The model under review builds one solid part; all positions refer to its coordinate system, in mm. A direction names the side the tool comes from. Give positions to 0.01 mm unless a question says otherwise; leave off trailing zeros. Order: outer loops, then holes, each group sorted by start corner. A loop starts at its lowest first (then second) coordinate and runs counter-clockwise, first axis right, second up. Notation, with made-up numbers: (0.25, 4.25) - (43.25, 4.25) arc R30 ccw to (43.25, 39.25) - close; hole circle Ø5 at (-4.5, -18.5). An arc over 180 degrees is marked (long way). Use a Markdown table: item, result. Add a question column.
```python
from build123d import *

# Parameters (mm, degrees)
F3_R     = 15
F3_R_2   = 7.5
F3_R_3   = 4.9
F4_DEPTH = 2
F5_DEPTH = 6
F6_DEPTH = 12.5


with BuildPart() as f4:
    # F3 (on Top) → F4 (new body)
    with BuildSketch(Plane.XY):
        Circle(F3_R)
        Circle(F3_R_2, mode=Mode.SUBTRACT)
        Circle(F3_R_2)
        Circle(F3_R_3, mode=Mode.SUBTRACT)
        Circle(F3_R_3)
        with BuildLine():
            ThreePointArc((-2.2847319318, -2.45), (-3.35, 0), (-2.2847319318, 2.45))
            Line((-2.2847319318, 2.45), (2.2847319318, 2.45))
            ThreePointArc((2.2847319318, 2.45), (3.35, 0), (2.2847319318, -2.45))
            Line((2.2847319318, -2.45), (-2.2847319318, -2.45))
        make_face(mode=Mode.SUBTRACT)
    extrude(amount=F4_DEPTH)

    # F3 (on Top) → F5 (join)
    with BuildSketch(Plane.XY):
        Circle(F3_R_2)
        Circle(F3_R_3, mode=Mode.SUBTRACT)
        Circle(F3_R_3)
        with BuildLine():
            ThreePointArc((-2.2847319318, -2.45), (-3.35, 0), (-2.2847319318, 2.45))
            Line((-2.2847319318, 2.45), (2.2847319318, 2.45))
            ThreePointArc((2.2847319318, 2.45), (3.35, 0), (2.2847319318, -2.45))
            Line((2.2847319318, -2.45), (-2.2847319318, -2.45))
        make_face(mode=Mode.SUBTRACT)
    extrude(amount=F5_DEPTH)

    # F3 (on Top) → F6 (join)
    with BuildSketch(Plane.XY):
        Circle(F3_R_3)
        with BuildLine():
            ThreePointArc((-2.2847319318, -2.45), (-3.35, 0), (-2.2847319318, 2.45))
            Line((-2.2847319318, 2.45), (2.2847319318, 2.45))
            ThreePointArc((2.2847319318, 2.45), (3.35, 0), (2.2847319318, -2.45))
            Line((2.2847319318, -2.45), (-2.2847319318, -2.45))
        make_face(mode=Mode.SUBTRACT)
    extrude(amount=F6_DEPTH)

    # F7 (on Front) → F8 (revolve)
    with BuildSketch(Plane.XZ):
        Polygon((5.15, 11.75), (4.9, 12.5), (4.9, 11), align=None)
    revolve(axis=Axis((0, 0, 8.7542282417), (0, 0, 1)))


solid = f4.part
```
Q1. Draft analysis for pull direction Z (two halves, no side actions). For faces 3 (the flat face through (0, -3, 12.5)), 4 (the flat face through (0, 2.45, 6)), 5 (the flat face through (0, -3, 0)), 6 (the cylindrical face through (-1.062, -4.783, 8.465)), state which applies: pulls with the +Z half, pulls with the -Z half, needs draft (parallel to the pull), parting line crosses it, or undercut.
Q2. Clearance check with flat-ended pins moving along their axes: P1, Ø1.5, axis at x = -1, z = 5.5, coming from the +Y side; P2, Ø8, axis at x = -11.5, y = -11, coming from the +Z side; P3, Ø12, axis at x = 1, y = 2, coming from the +Z side; P4, Ø10, axis at x = -11.5, y = -4.5, coming from the +Z side. State where each tip first meets the part, or that it passes through.
Q3. Wall thickness on probe 1 along Z at (x, y) = (-2.25, 9.75); probe 2 along X at (y, z) = (-2, 8.75); probe 3 along Y at (x, z) = (-2.25, 5.75): over which ranges is each line inside the solid? List them lowest first.
Q4. We need section A-A (y = 0). Write out the cut boundary in (x, z), plus the area to 3 significant figures.
Q5. We need section D-D (z = 10.25). Write out the cut boundary in (x, y).
Q6. We need section C-C (x = 0). Write out the cut boundary in (y, z).
Q7. We need section B-B (z = 3.5). Write out the cut boundary in (x, y).
Q8. Machinability: for faces 1 (the cylindrical face through (-3.35, -0.04, 6.16)), 2 (the cylindrical face through (-7.493, 0.33, 3.972)), which of the approach directions +Z, -Z, +X, -X, +Y, -Y give a long, thin tool a straight path to every point of the face, cutting with its end or side? Answer none if there is none.
Here are the results:
| question | item | result |
|---|---|---|
| 1 | face 3 | pulls with the +Z half |
| 1 | face 4 | needs draft |
| 1 | face 5 | pulls with the -Z half |
| 1 | face 6 | undercut |
| 2 | P1 | y = 7.5 |
| 2 | P2 | z = 2 |
| 2 | P3 | z = 12.5 |
| 2 | P4 | z = 6 |
| 3 | probe 1 | 0 to 2 |
| 3 | probe 2 | -4.47 to -2.69, 2.69 to 4.47 |
| 3 | probe 3 | -7.15 to -2.45, 2.45 to 7.15 |
| 4 | outline | (-15, 0) - (-3.35, 0) - (-3.35, 12.5) - (-4.9, 12.5) - (-5.15, 11.75) - (-4.9, 11) - (-4.9, 6) - (-7.5, 6) - (-7.5, 2) - (-15, 2) - close; (3.35, 0) - (15, 0) - (15, 2) - (7.5, 2) - (7.5, 6) - (4.9, 6) - (4.9, 11) - (5.15, 11.75) - (4.9, 12.5) - (3.35, 12.5) - close |
| 4 | area | 100 mm2 |
| 5 | outline | circle Ø9.8 at (0, 0); hole (-2.28, -2.45) - (2.28, -2.45) arc R3.35 ccw to (2.28, 2.45) - (-2.28, 2.45) arc R3.35 ccw to start |
| 6 | outline | (-15, 0) - (-2.45, 0) - (-2.45, 12.5) - (-4.9, 12.5) - (-5.15, 11.75) - (-4.9, 11) - (-4.9, 6) - (-7.5, 6) - (-7.5, 2) - (-15, 2) - close; (2.45, 0) - (15, 0) - (15, 2) - (7.5, 2) - (7.5, 6) - (4.9, 6) - (4.9, 11) - (5.15, 11.75) - (4.9, 12.5) - (2.45, 12.5) - close |
| 7 | outline | circle Ø15 at (0, 0); hole (-2.28, -2.45) - (2.28, -2.45) arc R3.35 ccw to (2.28, 2.45) - (-2.28, 2.45) arc R3.35 ccw to start |
| 8 | face 1 | +Z, -Z |
| 8 | face 2 | +Z |
